```python
from build123d import *

# Parameters (mm, degrees)
F0_W     = 21.03374
F0_H     = 6.19252
F1_DEPTH = 3.175
F2_W     = 1.27
F2_H     = 1.27
F3_DEPTH = 0.635
F5_W     = 0.762
F5_H     = 0.508
F6_DEPTH = 25.4
F7_R     = 0.254


with BuildPart() as f1:
    # F0 (on Top) → F1 (new body)
    with BuildSketch(Plane.XY):
        with Locations((1.38811, -1.27)):
            Rectangle(F0_W, F0_H)
    extrude(amount=F1_DEPTH)

    # F2 (on Top) → F3 (join)
    with BuildSketch(Plane.XY):
        with Locations((-6.95198, 2.46126)):
            Rectangle(F2_W, F2_H)
        with Locations((-4.56946, 2.46126)):
            Rectangle(F2_W, F2_H)
        with Locations((-2.18694, 2.46126)):
            Rectangle(F2_W, F2_H)
        with Locations((0.19558, 2.46126)):
            Rectangle(F2_W, F2_H)
        with Locations((2.5781, 2.46126)):
            Rectangle(F2_W, F2_H)
        with Locations((4.96062, 2.46126)):
            Rectangle(F2_W, F2_H)
        with Locations((7.34314, 2.46126)):
            Rectangle(F2_W, F2_H)
        with Locations((-6.95198, -5.00126)):
            Rectangle(F2_W, F2_H)
        with Locations((-4.56946, -5.00126)):
            Rectangle(F2_W, F2_H)
        with Locations((-2.18694, -5.00126)):
            Rectangle(F2_W, F2_H)
        with Locations((0.19558, -5.00126)):
            Rectangle(F2_W, F2_H)
        with Locations((2.5781, -5.00126)):
            Rectangle(F2_W, F2_H)
        with Locations((4.96062, -5.00126)):
            Rectangle(F2_W, F2_H)
        with Locations((7.34314, -5.00126)):
            Rectangle(F2_W, F2_H)
        with Locations((9.72566, 2.46126)):
            Rectangle(F2_W, F2_H)
        with Locations((9.72566, -5.00126)):
            Rectangle(F2_W, F2_H)
    extrude(amount=F3_DEPTH)

    # F5 (on face) → F6 (cut)
    with BuildSketch(Plane(origin=(-9.12876, 0, 0), x_dir=(0, -1, 0), z_dir=(-1, 0, 0))):
        with Locations((-1.44526, 2.921)):
            Rectangle(F5_W, F5_H)
        with Locations((3.98526, 2.921)):
            Rectangle(F5_W, F5_H)
    extrude(amount=-F6_DEPTH, mode=Mode.SUBTRACT)

    # F7
    f7_edges = [f1.edges().sort_by_distance(p)[0] for p in [
        (1.38811, 1.82626, 2.667),
        (1.38811, 1.06426, 3.175),
        (1.38811, -3.60426, 3.175),
        (1.38811, -4.36626, 2.667),
        (-9.12876, -1.27, 3.175),
        (-9.12876, -3.60426, 2.921),
        (-9.12876, -3.98526, 2.667),
        (-9.12876, -4.36626, 1.3335),
        (-9.12876, 1.44526, 2.667),
        (-9.12876, 1.06426, 2.921),
        (-9.12876, 1.82626, 1.3335),
        (11.90498, -4.36626, 1.3335),
        (11.90498, -3.98526, 2.667),
        (11.90498, -3.60426, 2.921),
        (11.90498, -1.27, 3.175),
        (11.90498, 1.06426, 2.921),
        (11.90498, 1.44526, 2.667),
        (11.90498, 1.82626, 1.3335),
    ]]
    fillet(f7_edges, radius=F7_R)


solid = f1.part
```
Geometry check sheet. Reference: the model listing, model coordinates, mm. A direction names the side the tool comes from. Give positions to 0.01 mm unless a question says otherwise; leave off trailing zeros. Order: outer loops, then holes, each group sorted by start corner. A loop starts at its lowest first (then second) coordinate and runs counter-clockwise, first axis right, second up. Notation, with made-up numbers: (84.5, -6) - (136.5, -6) arc R23 cw to (136.5, 9) - close; hole circle Ø7 at (49, -39). An arc over 180 degrees is marked (long way). Answer in a Markdown table with one row per item. Add a question column.
Q1. Cross-section at B-B, the plane z = 1.9. Enter the section's corners in (x, y).
Q2. Gauge pin test, flat ends, axial feed: pin 1 (0.6 mm diameter, centred on x = 10, y = -5, fed in from +Z) (3 decimals); pin 2 (0.7 mm diameter, centred on y = 2.5, z = 0.5, fed in from +X); pin 3 (1 mm diameter, centred on x = -4.5, y = 2, fed in from +Z); pin 4 (3 mm diameter, centred on x = 0.5, y = -1, fed in from -Z). Record the tip position at first contact, or that the pin passes through.
Q3. Mould release check, pull along X, two halves, no side actions. Record for faces 1 (the flat face through (-9.129, -1, 1)), 2 (the flat face through (1, 1.826, 1)), 3 (the flat face through (11.905, -1, 1)), 4 (the flat face through (10, -5, 0.635)): pulls with the +X half, pulls with the -X half, needs draft (parallel to the pull), parting line crosses it, or undercut.
Q4. Tool access check on faces 5 (the flat face through (10, 2, 0.635)), 6 (the flat face through (1, -1, 3.175)), 7 (the flat face through (-2, -5, 0.635)). Record the directions out of +Z, -Z, +X, -X, +Y, -Y that give a thin tool (end or side, any length) a straight path to the whole face; none if there is none.
Q5. Cross-section at C-C, the plane x = 8.75. Enter the section's corners in (y, z) (3 decimals).
Q6. Cross-section at A-A, the plane y = -5. Count the separate pieces of the cut face and the enclosed holes in it, then the cut area to 3 significant figures.
Q7. Material ranges on probe 1 along Y at (x, z) = (9.25, 1.6); probe 2 along Z at (x, y) = (-4.75, 2.25) (3 decimals); probe 3 along Z at (x, y) = (2.75, 1.5), recorded low to high. Write a range as from..to.
Q8. Cross-section at D-D, the plane x = -0.25. Enter the section's corners in (y, z) (3 decimals).
Check values:
| question | item | result |
|---|---|---|
| 1 | outline | (-9.13, -4.11) arc R0.25 ccw to (-8.87, -4.37) - (11.65, -4.37) arc R0.25 ccw to (11.9, -4.11) - (11.9, 1.57) arc R0.25 ccw to (11.65, 1.83) - (-8.87, 1.83) arc R0.25 ccw to (-9.13, 1.57) - close |
| 2 | pin 1 | stops at z = 0.635 |
| 2 | pin 2 | stops at x = 10.36 |
| 2 | pin 3 | stops at z = 2.67 |
| 2 | pin 4 | stops at z = 0 |
| 3 | face 1 | pulls with the -X half |
| 3 | face 2 | undercut |
| 3 | face 3 | pulls with the +X half |
| 3 | face 4 | needs draft |
| 4 | face 5 | +Z, +X, -X, +Y |
| 4 | face 6 | +Z, +X, -X, +Y, -Y |
| 4 | face 7 | +Z, +X, -X, -Y |
| 5 | outline | (-4.366, 0) - (1.826, 0) - (1.826, 2.413) arc R0.254 ccw to (1.572, 2.667) - (1.064, 2.667) - (1.064, 2.921) arc R0.254 ccw to (0.81, 3.175) - (-3.35, 3.175) arc R0.254 ccw to (-3.604, 2.921) - (-3.604, 2.667) - (-4.112, 2.667) arc R0.254 ccw to (-4.366, 2.413) - close |
| 6 | separate pieces | 8 |
| 6 | enclosed holes | 0 |
| 6 | area | 6.45 mm^2 |
| 7 | probe 1 | y = -4.37..1.83 |
| 7 | probe 2 | z = 0..0.635 |
| 7 | probe 3 | z = 0..2.67 |
| 8 | outline | (-5.636, 0) - (3.096, 0) - (3.096, 0.635) - (1.826, 0.635) - (1.826, 2.413) arc R0.254 ccw to (1.572, 2.667) - (1.064, 2.667) - (1.064, 2.921) arc R0.254 ccw to (0.81, 3.175) - (-3.35, 3.175) arc R0.254 ccw to (-3.604, 2.921) - (-3.604, 2.667) - (-4.112, 2.667) arc R0.254 ccw to (-4.366, 2.413) - (-4.366, 0.635) - (-5.636, 0.635) - close |
